The model under review builds one solid part; all positions refer to its coordinate system, in mm. Face numbers are marked on the shaded views. A direction names the side the tool comes from. Give positions to 0.01 mm unless a question says otherwise; leave off trailing zeros. Loops run counter-clockwise (first coordinate to the right, second up) from the corner with the lowest first, then second, coordinate; pieces in that order, holes last. Notation, with made-up numbers: (85.5, 32.25) -> (101.5, 32.25) arc R7 ccw to (101.5, 38.25) -> close; hole circle Ø6 at (61, -29.5). An arc over 180 degrees is marked (long way). Write each question's results on one line, items separated by ' | '. Start each with the question number.
Q1. Machinability: for the marked faces 1, 2 and 3, which of the approach directions +Z, -Z, +X, -X, +Y, -Y give a long, thin tool a straight path to every point of the face, cutting with its end or side? Answer none if there is none.
Q2. We need section A-A (x = 0). Write out the cut boundary in (y, z).
Q3. Mouldability with a two-part tool opening along Y and no side actions: class the marked faces 4, 5 and 6 as released by +Y, released by -Y, zero draft, split by the parting line, or undercut.
Q4. Insertion check: pin 1 Ø12 at (x, y) = (-17, 85) entering from -Z; pin 2 Ø19 at (x, z) = (24.5, -24) entering from -Y; pin 3 Ø5 at (x, z) = (8, 4) entering from +Y. Each pin has a flat end and moves straight along its axis. Give the tip position at first contact, or say it passes through.
Q5. We need section C-C (y = -49.5). Write out the cut boundary in (x, z), plus the area to 3 significant figures.
Q6. Wall thickness on L1, parallel to Z at x = 5, y = 0; L2, parallel to Y at x = -6, z = -19.05; L3, parallel to Z at x = -37, y = 2: over which ranges is each line inside the solid? List them lowest first. Write a range as [from, to].
Q7. We need section B-B (x = 28.5). Write out the cut boundary in (y, z), plus the area to 3 significant figures.
Q8. We need section D-D (y = -93). Write out the cut boundary in (x, z), plus the area to 3 significant figures.
from build123d import *

# Parameters (mm, degrees)
F1_DEPTH = 12.7
F2_W     = 101.6
F2_H     = 88.9
F3_DEPTH = 38.1
F5_D     = 25.4
F5_DEPTH = 76.2
F5_TIP   = 7.6309298617
F6_W     = 6.35
F6_H     = 25.4
F7_DEPTH = 6.35
F8_W     = 88.9
F8_H     = 27.94
F9_DEPTH = 6.35


with BuildPart() as f1:
    # F0 (on Top) → F1 (new body)
    with BuildSketch(Plane.XY):
        with BuildLine():
            Line((-50.8, 88.9), (-50.8, -88.9))
            ThreePointArc((-50.8, -88.9), (0, -139.7), (50.8, -88.9))
            Line((50.8, -88.9), (50.8, 88.9))
            ThreePointArc((50.8, 88.9), (0, 139.7), (-50.8, 88.9))
        make_face()
    extrude(amount=F1_DEPTH)

    # F2 (on face) → F3 (join)
    with BuildSketch(Plane(origin=(0, 0, 0), x_dir=(1, 0, 0), z_dir=(0, 0, -1))):
        Rectangle(F2_W, F2_H)
    extrude(amount=F3_DEPTH)

    # F5
    with Locations(Plane(origin=(-50.8, 0, 0), x_dir=(0, -1, 0), z_dir=(-1, 0, 0))):
        with Locations((0, -19.05)):
            Hole(F5_D / 2, depth=F5_DEPTH)
            with Locations((0, 0, -(F5_DEPTH + F5_TIP / 2))):  # 118° drill point
                Cone(0, F5_D / 2, F5_TIP, mode=Mode.SUBTRACT)

    # F6 (on face) → F7 (cut)
    with BuildSketch(Plane.XY.offset(12.7)):
        with Locations((-41.275, 0)):
            Rectangle(F6_W, F6_H)
        with Locations((41.275, 0)):
            Rectangle(F6_W, F6_H)
    extrude(amount=-F7_DEPTH, mode=Mode.SUBTRACT)

    # F8 (on face) → F9 (cut)
    with BuildSketch(Plane(origin=(0, 0, 0), x_dir=(1, 0, 0), z_dir=(0, 0, -1))):
        Rectangle(F8_W, F8_H)
    extrude(amount=-F9_DEPTH, mode=Mode.SUBTRACT)


solid = f1.part
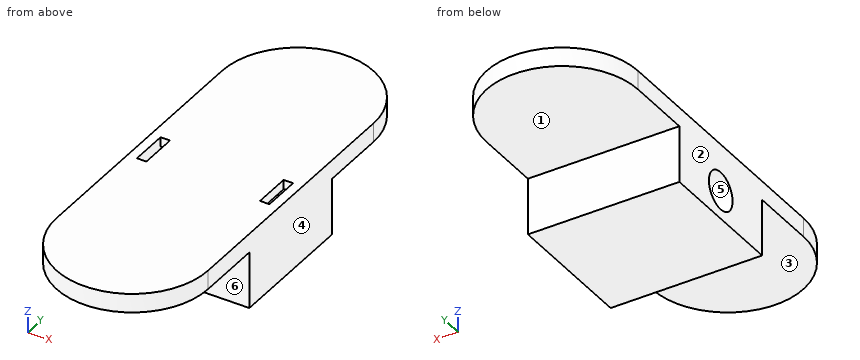
Output:
1) face 1: -Z, +X, -X, +Y | face 2: +Z, -Z, -X, +Y, -Y | face 3: -Z, +X, -X, -Y
2) outline: (-139.7, 0) -> (-44.45, 0) -> (-44.45, -38.1) -> (44.45, -38.1) -> (44.45, 0) -> (139.7, 0) -> (139.7, 12.7) -> (-139.7, 12.7) -> close; hole (-13.97, 0) -> (13.97, 0) -> (13.97, 6.35) -> (-13.97, 6.35) -> close; hole circle Ø25.4 at (0, -19.05)
3) face 4: zero draft | face 5: undercut | face 6: released by -Y
4) pin 1: z = 0 | pin 2: y = -44.45 | pin 3: y = 139.4
5) outline: (-50.8, 0) -> (50.8, 0) -> (50.8, 12.7) -> (-50.8, 12.7) -> close | area: 1,290 mm2
6) L1: [-38.1, -31.75], [-6.35, 0], [6.35, 12.7] | L2: [-44.45, -12.7], [12.7, 44.45] | L3: [-38.1, -31.59], [-6.51, 0], [6.35, 12.7]
7) outline: (-130.95, 0) -> (-44.45, 0) -> (-44.45, -38.1) -> (44.45, -38.1) -> (44.45, 0) -> (130.95, 0) -> (130.95, 12.7) -> (-130.95, 12.7) -> close; hole (-13.97, 0) -> (13.97, 0) -> (13.97, 6.35) -> (-13.97, 6.35) -> close; hole circle Ø15.08 at (0, -19.05) | area: 6,360 mm2
8) outline: (-50.63, 0) -> (50.63, 0) -> (50.63, 12.7) -> (-50.63, 12.7) -> close | area: 1,290 mm2
